```python
from build123d import *

# Parameters (mm, degrees)
CROQUIS2_W                         = 170
CROQUIS2_H                         = 90
SALIENTE_EXTRUIR1_DEPTH            = 23
REDONDEO1_R                        = 5
VACIADO1_T                         = -3
REDONDEO4_R                        = 2
CHAFL_N1_SIZE                      = 2
CORTAR_EXTRUIR1_REACH              = 179.353
CROQUIS3_W                         = 14
CROQUIS3_H                         = 19.902430744
CROQUIS3_W_2                       = 10
CROQUIS3_H_2                       = 25.118860909
REDONDEO2_R                        = 1
CROQUIS4_W                         = 18.994013978
CROQUIS4_H                         = 9.979905649
CORTAR_EXTRUIR2_DEPTH              = 99.234413522
REDONDEO3_R                        = 1
SELECCIONAR_OPERACIONES1_OUTLINE_W = 1.395184441
SELECCIONAR_OPERACIONES1_OUTLINE_H = 17.925
SELECCIONAR_OPERACIONES1_DEPTH     = 2
SELECCIONAR_OPERACIONES1_DRAFT     = -3
SELECCIONAR_OPERACIONES1_2_DEPTH   = 2
SELECCIONAR_OPERACIONES1_2_DRAFT   = -3
TALADRO_DE_MARGEN_PARA_M41_D       = 4.5


# Read off the part's stored shape, not the designer's step: Saliente de montaje5, Seleccionar operaciones1
with BuildPart() as part:
    # Croquis2 → Saliente-Extruir1 (new body)
    with BuildSketch(Plane(origin=(0, 0, 0), x_dir=(1, 0, 0), z_dir=(0, 1, 0))):
        Rectangle(CROQUIS2_W, CROQUIS2_H)
    extrude(amount=SALIENTE_EXTRUIR1_DEPTH)

    # Redondeo1
    redondeo1_edges = [part.edges().sort_by_distance(p)[0] for p in [
        (85, 11.5, 45),
        (-85, 11.5, 45),
        (-85, 11.5, -45),
        (85, 11.5, -45),
    ]]
    fillet(redondeo1_edges, radius=REDONDEO1_R)

    # Vaciado1
    vaciado1_openings = [part.faces().sort_by_distance(p)[0] for p in [
        (0, 23, 0),
    ]]
    offset(amount=VACIADO1_T, openings=vaciado1_openings, kind=Kind.INTERSECTION)

    # Redondeo4
    redondeo4_edges = [part.edges().sort_by_distance(p)[0] for p in [
        (82, 3, 0),
        (0, 3, -42),
        (-82, 3, 0),
        (0, 3, 42),
        (81.414213562, 3, 41.414213562),
        (-81.414213562, 3, 41.414213562),
        (-81.414213562, 3, -41.414213562),
        (81.414213562, 3, -41.414213562),
    ]]
    fillet(redondeo4_edges, radius=REDONDEO4_R)

    # Chaflán1
    chafl_n1_edges = [part.edges().sort_by_distance(p)[0] for p in [
        (85, 0, 0),
        (0, 0, 45),
        (-85, 0, 0),
        (0, 0, -45),
        (-83.535533906, 0, 43.535533906),
        (-83.535533906, 0, -43.535533906),
        (83.535533906, 0, -43.535533906),
        (83.535533906, 0, 43.535533906),
    ]]
    chamfer(chafl_n1_edges, length=CHAFL_N1_SIZE)

    # Saliente de montaje5 outline → Saliente de montaje5 (revolve, cut)
    with BuildSketch(Plane(origin=(-54.53, 0, 24.462759338), x_dir=(1, 0, 0), z_dir=(0, 0, 1))):
        Polygon((2.128547792, 0), (2.076182597, 3), (0, 3), (0, 0), align=None)
    saliente_de_montaje5 = revolve(axis=Axis((-54.53, 0, 24.462759338), (0, 1, 0)), mode=Mode.SUBTRACT)

    # Saliente de montaje5 2 outline → Saliente de montaje5 2 (revolve)
    with BuildSketch(Plane(origin=(-54.53, 0, 24.462759338), x_dir=(1, 0, 0), z_dir=(0, 0, 1))):
        Polygon((4, 6), (2.587488664, 6), (2.5, 7), (1.6, 7), (1.6, 4.5), (2.05, 4.5), (2.076182597, 3), (4.262465991, 3), align=None)
    saliente_de_montaje5_2 = revolve(axis=Axis((-54.53, 0, 24.462759338), (0, 1, 0)))

    # Matriz de croquis1: Saliente de montaje5, Saliente de montaje5 2 at 8 more places
    with Locations((1.27, 0, -48.26), (52.07, 0, -33.02), (52.07, 0, -5.08), (82.55, 0, 0), (76.2, 0, -48.26), (111.63, 0, -26.46), (95.88, 0, -0.46), (127.38, 0, -0.46)):
        add(saliente_de_montaje5, mode=Mode.SUBTRACT)
        add(saliente_de_montaje5_2)

    # Croquis3 → Cortar-Extruir1 (cut, up to next)
    with BuildSketch(Plane.ZY.offset(85), mode=Mode.PRIVATE) as cortar_extruir1_sk1:
        with Locations((-11.097240662, 17.951215372)):
            Rectangle(CROQUIS3_W, CROQUIS3_H)
    cortar_extruir1_tool1 = extrude(cortar_extruir1_sk1.sketch, amount=-CORTAR_EXTRUIR1_REACH, mode=Mode.PRIVATE) & part.part
    # Croquis3 → Cortar-Extruir1 (cut, up to next)
    with BuildSketch(Plane.ZY.offset(85), mode=Mode.PRIVATE) as cortar_extruir1_sk2:
        with Locations((18.827759338, 20.559430454)):
            Rectangle(CROQUIS3_W_2, CROQUIS3_H_2)
    cortar_extruir1_tool2 = extrude(cortar_extruir1_sk2.sketch, amount=-CORTAR_EXTRUIR1_REACH, mode=Mode.PRIVATE) & part.part
    add(cortar_extruir1_tool1.solids().sort_by_distance((-85, 17.951215, -11.097241))[0], mode=Mode.SUBTRACT)
    add(cortar_extruir1_tool2.solids().sort_by_distance((-85, 20.55943, 18.827759))[0], mode=Mode.SUBTRACT)

    # Redondeo2
    redondeo2_edges = [part.edges().sort_by_distance(p)[0] for p in [
        (-83.5, 8, -4.097240662),
        (-83.5, 8, -18.097240662),
        (-83.5, 8, 23.827759338),
        (-83.5, 8, 13.827759338),
    ]]
    fillet(redondeo2_edges, radius=REDONDEO2_R)

    # Croquis4 → Cortar-Extruir2 (cut, through all)
    with BuildSketch(Plane(origin=(0, 3, 0), x_dir=(1, 0, 0), z_dir=(0, 1, 0))):
        with Locations((43.352971059, 18.87114604)):
            Rectangle(CROQUIS4_W, CROQUIS4_H)
    extrude(amount=-CORTAR_EXTRUIR2_DEPTH, mode=Mode.SUBTRACT)

    # Redondeo3
    redondeo3_edges = [part.edges().sort_by_distance(p)[0] for p in [
        (52.849978048, 1.5, -23.861098864),
        (52.849978048, 1.5, -13.881193215),
        (33.85596407, 1.5, -13.881193215),
        (33.85596407, 1.5, -23.861098864),
    ]]
    fillet(redondeo3_edges, radius=REDONDEO3_R)


with BuildPart() as seleccionar_operaciones1_tool:
    # Seleccionar operaciones1 outline → Seleccionar operaciones1 (with draft: the straight prism first)
    with BuildSketch(Plane(origin=(0, 21, 0), x_dir=(1, 0, 0), z_dir=(0, 1, 0))):
        with Locations((-84.30240778, -4.865259338)):
            Rectangle(SELECCIONAR_OPERACIONES1_OUTLINE_W, SELECCIONAR_OPERACIONES1_OUTLINE_H)
    extrude(amount=SELECCIONAR_OPERACIONES1_DEPTH)
    # Seleccionar operaciones1: the draft: its side faces are tilted about the plane it starts from
    seleccionar_operaciones1_sides = [seleccionar_operaciones1_tool.faces().sort_by_distance(p)[0] for p in [
        (-84.30240778, 22, 13.827759338),
        (-83.604815559, 22, 4.865259338),
        (-84.30240778, 22, -4.097240662),
        (-85, 22, 4.865259338),
    ]]
    draft(seleccionar_operaciones1_sides, Plane(origin=(0, 21, 0), x_dir=(1, 0, 0), z_dir=(0, 1, 0)), SELECCIONAR_OPERACIONES1_DRAFT)


with BuildPart() as part_1:
    add(part.part)

    # Seleccionar operaciones1: cut by seleccionar_operaciones1_tool
    add(seleccionar_operaciones1_tool.part, mode=Mode.SUBTRACT)


with BuildPart() as seleccionar_operaciones1_2_tool:
    # Seleccionar operaciones1 2 outline → Seleccionar operaciones1 2 (with draft: the straight prism first)
    with BuildSketch(Plane(origin=(0, 21, 0), x_dir=(1, 0, 0), z_dir=(0, 1, 0))):
        with BuildLine():
            Line((-83.604815559, -23.827759338), (-85, -23.827759338))
            Line((-85, -23.827759338), (-85, -40))
            ThreePointArc((-85, -40), (-83.535533906, -43.535533906), (-80, -45))
            Line((-80, -45), (80, -45))
            ThreePointArc((80, -45), (83.535533906, -43.535533906), (85, -40))
            Line((85, -40), (85, 40))
            ThreePointArc((85, 40), (83.535533906, 43.535533906), (80, 45))
            Line((80, 45), (-80, 45))
            ThreePointArc((-80, 45), (-83.535533906, 43.535533906), (-85, 40))
            Line((-85, 40), (-85, 18.097240662))
            Line((-85, 18.097240662), (-83.604815559, 18.097240662))
            Line((-83.604815559, 18.097240662), (-83.604815559, 40))
            ThreePointArc((-83.604815559, 40), (-82.548989526, 42.548989526), (-80, 43.604815559))
            Line((-80, 43.604815559), (80, 43.604815559))
            ThreePointArc((80, 43.604815559), (82.548989526, 42.548989526), (83.604815559, 40))
            Line((83.604815559, 40), (83.604815559, -40))
            ThreePointArc((83.604815559, -40), (82.548989526, -42.548989526), (80, -43.604815559))
            Line((80, -43.604815559), (-80, -43.604815559))
            ThreePointArc((-80, -43.604815559), (-82.548989526, -42.548989526), (-83.604815559, -40))
            Line((-83.604815559, -40), (-83.604815559, -23.827759338))
        make_face()
    extrude(amount=SELECCIONAR_OPERACIONES1_2_DEPTH)
    # Seleccionar operaciones1 2: the draft: its side faces are tilted about the plane it starts from
    seleccionar_operaciones1_2_sides = [seleccionar_operaciones1_2_tool.faces().sort_by_distance(p)[0] for p in [
        (-82.548989526, 22, 42.548989526),
        (-83.604815559, 22, 31.913879669),
        (-84.30240778, 22, 23.827759338),
        (-85, 22, 31.913879669),
        (-83.535533906, 22, 43.535533906),
        (0, 22, 45),
        (83.535533906, 22, 43.535533906),
        (85, 22, 0),
        (83.535533906, 22, -43.535533906),
        (0, 22, -45),
        (-83.535533906, 22, -43.535533906),
        (-85, 22, -29.048620331),
        (-84.30240778, 22, -18.097240662),
        (-83.604815559, 22, -29.048620331),
        (-82.548989526, 22, -42.548989526),
        (0, 22, -43.604815559),
        (82.548989526, 22, -42.548989526),
        (83.604815559, 22, 0),
        (82.548989526, 22, 42.548989526),
        (0, 22, 43.604815559),
    ]]
    draft(seleccionar_operaciones1_2_sides, Plane(origin=(0, 21, 0), x_dir=(1, 0, 0), z_dir=(0, 1, 0)), SELECCIONAR_OPERACIONES1_2_DRAFT)


with BuildPart() as part_2:
    add(part_1.part)

    # Seleccionar operaciones1 2: cut by seleccionar_operaciones1_2_tool
    add(seleccionar_operaciones1_2_tool.part, mode=Mode.SUBTRACT)

    # Taladro de margen para M41 (through all)
    with Locations(Plane(origin=(0, 3, 0), x_dir=(1, 0, 0), z_dir=(0, 1, 0))):
        with Locations((0, 0), (40, -32.5), (-40, 32.5), (-40, -32.5), (40, 32.5)):
            Hole(TALADRO_DE_MARGEN_PARA_M41_D / 2)


solid = part_2.part
```
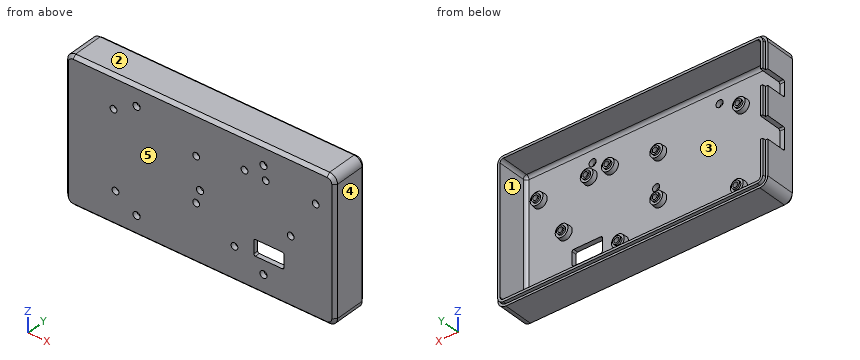
Read the model definition and answer for the solid it produces. Units are mm, in the model's axes. Face numbers are marked on the shaded views. A direction names the side the tool comes from. Coordinates: 2 decimals unless noted, no trailing zeros. Loops run counter-clockwise (first coordinate to the right, second up) from the corner with the lowest first, then second, coordinate; pieces in that order, holes last. Notation, with made-up numbers: (36.25, 3) -> (47.25, 3) arc R22 ccw to (47.25, 27) -> close; hole circle Ø6 at (-36.5, -18.75). An arc over 180 degrees is marked (long way). Return JSON: item names as keys, results as strings.
Item 1: Find section C-C (x = -40). Determine the outline of the cut face in (y, z).
Answers:
{"outline": "(0, -43) -> (2, -45) -> (21, -45) -> (21, -43.6) -> (23, -43.5) -> (23, -42) -> (5, -42) arc R2 cw to (3, -40) -> (3, -34.75) -> (0, -34.75) -> close; (0, -30.25) -> (3, -30.25) -> (3, 30.25) -> (0, 30.25) -> close; (0, 34.75) -> (3, 34.75) -> (3, 40) arc R2 cw to (5, 42) -> (23, 42) -> (23, 43.5) -> (21, 43.6) -> (21, 45) -> (2, 45) -> (0, 43) -> close"}
Item 2: Find section D-D (x = 50). Determine the outline of the cut face in (y, z), plus the area to 3 significant figures.
Answers:
{"outline": "(0, -43) -> (2, -45) -> (21, -45) -> (21, -43.6) -> (23, -43.5) -> (23, -42) -> (5, -42) arc R2 cw to (3, -40) -> (3, -23.86) -> (0, -23.86) -> close; (0, -13.88) -> (3, -13.88) -> (3, 40) arc R2 cw to (5, 42) -> (23, 42) -> (23, 43.5) -> (21, 43.6) -> (21, 45) -> (2, 45) -> (0, 43) -> close", "area": "352 mm2"}
Item 3: Find section B-B (z = -32.5). Determine the outline of the cut face in (x, y), plus the area to 3 significant figures.
Answers:
{"outline": "(-85, 2) -> (-83, 0) -> (-42.25, 0) -> (-42.25, 3) -> (-80, 3) arc R2 cw to (-82, 5) -> (-82, 23) -> (-83.5, 23) -> (-83.6, 21) -> (-85, 21) -> close; (-37.75, 0) -> (37.75, 0) -> (37.75, 3) -> (-37.75, 3) -> close; (42.25, 0) -> (83, 0) -> (85, 2) -> (85, 21) -> (83.6, 21) -> (83.5, 23) -> (82, 23) -> (82, 5) arc R2 cw to (80, 3) -> (42.25, 3) -> close", "area": "595 mm2"}
Item 4: For the marked faces 1 and 2, determine the directions among +Z, -Z, +X, -X, +Y, -Y from which every point of the face is accessible in a straight line to the end or side of a thin tool.
Answers:
{"face 1": "+Y", "face 2": "+Z, +X, -X, +Y, -Y"}
Item 5: Find the intervals of material crossed by probe 1 along X at (y, z) = (12, -18.5); probe 2 along Z at (x, y) = (29, 20.25); probe 3 along Z at (x, y) = (72.85, 6.55), in increasing order.
Answers:
{"probe 1": "x = -85 to -82, 82 to 85", "probe 2": "z = -45 to -42, 42 to 45", "probe 3": "z = -45 to -42, 21.46 to 22.4, 25.6 to 26.54, 42 to 45"}
Item 6: Flat-ended cylindrical pins translate along their axes: P1, Ø6.5, axis at x = 22, z = -25, coming from the +Y side; P2, Ø2.5, axis at x = -40, z = 32.5, coming from the -Y side; P3, Ø24, axis at x = 33, z = 8, coming from the +Y side; P4, Ø3.5, axis at y = 1.5, z = -17.5, coming from the +X side. Find the tip coordinate at first contact, or state that the pin passes through.
Answers:
{"P1": "stops at y = 7", "P2": "passes through", "P3": "stops at y = 3", "P4": "stops at x = 85"}
Item 7: Find section A-A (y = 16.25). Determine the outline of the cut face in (x, z), plus the area to 3 significant figures.
Answers:
{"outline": "(-85, -40) arc R5 ccw to (-80, -45) -> (80, -45) arc R5 ccw to (85, -40) -> (85, 40) arc R5 ccw to (80, 45) -> (-80, 45) arc R5 ccw to (-85, 40) -> (-85, 23.83) -> (-82, 23.83) -> (-82, 40) arc R2 cw to (-80, 42) -> (80, 42) arc R2 cw to (82, 40) -> (82, -40) arc R2 cw to (80, -42) -> (-80, -42) arc R2 cw to (-82, -40) -> (-82, -18.1) -> (-85, -18.1) -> close; (-85, -4.1) -> (-82, -4.1) -> (-82, 13.83) -> (-85, 13.83) -> close", "area": "1,430 mm2"}
Item 8: For a pull along X with two mould halves and no side action, classify the marked faces 3, 4 and 5 as +X half, -X half, draft (parallel to the pull), parting line (faces both ways), or undercut.
Answers:
{"face 3": "undercut", "face 4": "+X half", "face 5": "draft"}
